```python
from build123d import *

# Parameters (mm, degrees)
SKETCH1_W           = 200
SKETCH1_H           = 100
BOSS_EXTRUDE1_DEPTH = 50
SKETCH3_W           = 198.6
SKETCH3_H           = 98.6
CUT_EXTRUDE1_DEPTH  = 49.3
SKETCH4_W           = 54.3
SKETCH4_H           = 98.6
BOSS_EXTRUDE2_DEPTH = 0.7
SKETCH2_R           = 4.5
SKETCH2_R_2         = 1.5
CUT_EXTRUDE2_DEPTH  = 230.128784748
SKETCH6_R           = 1.5
CUT_EXTRUDE3_DEPTH  = 0.7
SKETCH7_R           = 1.5
CUT_EXTRUDE4_DEPTH  = 0.7
CUT_EXTRUDE6_REACH  = 214.132
SKETCH8_R           = 1.21


with BuildPart() as part:
    # Sketch1 → Boss-Extrude1 (new body)
    with BuildSketch(Plane(origin=(0, 0, 0), x_dir=(1, 0, 0), z_dir=(0, 1, 0))):
        with Locations((100, 0)):
            Rectangle(SKETCH1_W, SKETCH1_H)
    extrude(amount=BOSS_EXTRUDE1_DEPTH)

    # Sketch3 → Cut-Extrude1 (cut)
    with BuildSketch(Plane.XZ):
        with Locations((100, 0)):
            Rectangle(SKETCH3_W, SKETCH3_H)
    extrude(amount=-CUT_EXTRUDE1_DEPTH, mode=Mode.SUBTRACT)

    # Sketch4 → Boss-Extrude2 (add)
    with BuildSketch(Plane.XZ):
        with Locations((172.15, 0)):
            Rectangle(SKETCH4_W, SKETCH4_H)
    extrude(amount=-BOSS_EXTRUDE2_DEPTH)

    # Sketch2 → Cut-Extrude2 (cut, through all)
    with BuildSketch(Plane.XY.offset(50)):
        with Locations((50, 14)):
            Circle(SKETCH2_R)
        with Locations((50, 4)):
            Circle(SKETCH2_R_2)
        with Locations((50, 24)):
            Circle(SKETCH2_R_2)
    extrude(amount=-CUT_EXTRUDE2_DEPTH, mode=Mode.SUBTRACT)

    # Sketch6 → Cut-Extrude3 (cut)
    with BuildSketch(Plane.XY.offset(50)):
        with Locations((4.6, 45)):
            Circle(SKETCH6_R)
        with Locations((4.6, 35)):
            Circle(SKETCH6_R)
        with Locations((54.1, 45)):
            Circle(SKETCH6_R)
        with Locations((54.1, 35)):
            Circle(SKETCH6_R)
        with Locations((69.1, 45)):
            Circle(SKETCH6_R)
        with Locations((69.1, 35)):
            Circle(SKETCH6_R)
    extrude(amount=-CUT_EXTRUDE3_DEPTH, mode=Mode.SUBTRACT)

    # Sketch7 → Cut-Extrude4 (cut)
    with BuildSketch(Plane.ZY):
        with Locations((42, 45)):
            Circle(SKETCH7_R)
        with Locations((42, 35)):
            Circle(SKETCH7_R)
    extrude(amount=-CUT_EXTRUDE4_DEPTH, mode=Mode.SUBTRACT)

    # Sketch8 → Cut-Extrude6 (cut, up to next)
    with BuildSketch(Plane.XZ, mode=Mode.PRIVATE) as cut_extrude6_sk1:
        with Locations(Location((160, 8.45, 0), (0, 0, 270))):
            Circle(SKETCH8_R)
    cut_extrude6_tool1 = extrude(cut_extrude6_sk1.sketch, amount=-CUT_EXTRUDE6_REACH, mode=Mode.PRIVATE) & part.part
    # Sketch8 → Cut-Extrude6 (cut, up to next)
    with BuildSketch(Plane.XZ, mode=Mode.PRIVATE) as cut_extrude6_sk2:
        with Locations(Location((160, -7.05, 0), (0, 0, 270))):
            Circle(SKETCH8_R)
    cut_extrude6_tool2 = extrude(cut_extrude6_sk2.sketch, amount=-CUT_EXTRUDE6_REACH, mode=Mode.PRIVATE) & part.part
    add(cut_extrude6_tool1.solids().sort_by_distance((160, 0, 8.45))[0], mode=Mode.SUBTRACT)
    add(cut_extrude6_tool2.solids().sort_by_distance((160, 0, -7.05))[0], mode=Mode.SUBTRACT)


solid = part.part
```
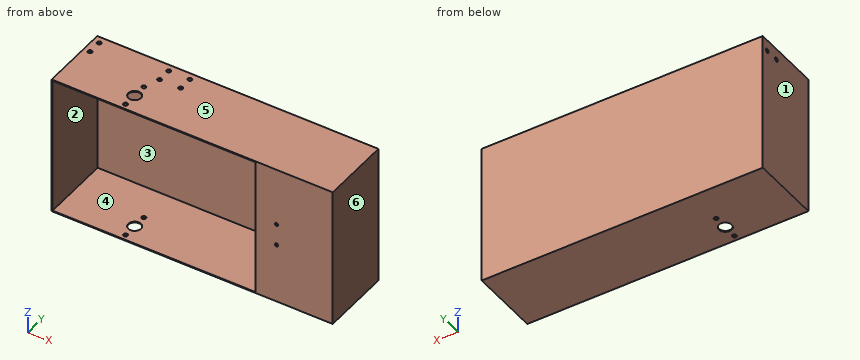
Work out the finished part from the listing and answer in its coordinate system (mm). Face numbers are marked on the shaded views. A direction names the side the tool comes from. Coordinates: 2 decimals unless noted, no trailing zeros. Loops run counter-clockwise (first coordinate to the right, second up) from the corner with the lowest first, then second, coordinate; pieces in that order, holes last. Notation, with made-up numbers: (42, -8.75) -> (56, -8.75) arc R28 ccw to (56, 20.25) -> close; hole circle Ø1 at (-5, 20.5). An arc over 180 degrees is marked (long way). Answer as CSV lines item,"result".
Q1. Each of these flat-tipped pins is pushed along its axis until it touches: pin 1 (1.5 mm diameter, centred on x = 144, z = -6.5, fed in from -Y); pin 2 (2.5 mm diameter, centred on y = 45, z = 42, fed in from -X). Where does it stop, or does it pass through?
Findings:
pin 1,"stops at y = 49.3"
pin 2,"stops at x = 199.3"
Q2. For a pull along Z with two mould halves and no side action, classify the marked faces 4, 5 and 6 as +Z half, -Z half, draft (parallel to the pull), parting line (faces both ways), or undercut.
Findings:
face 4,"undercut"
face 5,"+Z half"
face 6,"draft"
Q3. The part is cut by section B-B on z = -43. Write down the section's boundary in (x, y).
Findings:
outline,"(0, 0) -> (0.7, 0) -> (0.7, 49.3) -> (199.3, 49.3) -> (199.3, 0.7) -> (145, 0.7) -> (145, 0) -> (200, 0) -> (200, 50) -> (0, 50) -> close"
Q4. A tool of negligible diameter and unlimited length cuts with its end or side. For the marked faces 1, 2 and 3, from which of +Z, -Z, +X, -X, +Y, -Y can it reach the whole face along a straight path? Write none if from no direction.
Findings:
face 1,"+Z, -Z, -X, +Y, -Y"
face 2,"-Y"
face 3,"none"
Q5. The part is cut by section A-A on y = 30.5. Write down the section's boundary in (x, z).
Findings:
outline,"(0, -50) -> (200, -50) -> (200, 50) -> (0, 50) -> close; hole (0.7, -49.3) -> (199.3, -49.3) -> (199.3, 49.3) -> (0.7, 49.3) -> close"
Q6. Find the intervals of material crossed by probe 1 along Z at (x, y) = (160, 0.45); probe 2 along Y at (x, z) = (50, -49.5); probe 3 along X at (y, z) = (4, 49), in increasing order.
Findings:
probe 1,"z = -50 to -8.26, -5.84 to 7.24, 9.66 to 50"
probe 2,"y = 0 to 2.5, 5.5 to 9.5, 18.5 to 22.5, 25.5 to 50"
probe 3,"x = 0 to 0.7, 199.3 to 200"
Q7. The part is cut by section C-C on x = 137. Write down the section's boundary in (y, z), and give its area (3 significant figures).
Findings:
outline,"(0, -50) -> (50, -50) -> (50, 50) -> (0, 50) -> (0, 49.3) -> (49.3, 49.3) -> (49.3, -49.3) -> (0, -49.3) -> close"
area,"139 mm²"
